Part print with two shaded views. Sizes in mm from the minimum x, y, z corner. A direction names the side the tool comes from. Round coordinates to 2 decimals unless told otherwise and drop trailing zeros. Order: outer loops, then holes, each group sorted by start corner. A loop starts at its lowest first (then second) coordinate and runs counter-clockwise, first axis right, second up. Notation, with made-up numbers: M 83.5,33 L 131.5,33 A12 cw 131.5,37 Z; hole C 37.5,83 d3. An arc over 180 degrees is marked long. Return JSON: item names as keys, results as strings. Group by question number.
Item 1: Pull direction X, two halves, no side cores. Call the marked faces 1, 2 and 3: pulls with the +X half, pulls with the -X half, needs draft (parallel to the pull), parting line crosses it, or undercut.
Item 2: Slice it at D-D on y = 24. Write the cut outline in (x, z) (3 decimals), then the cut area to 3 significant figures.
Item 3: Pin check, flat tips, straight feed: pin 1 Ø3.5 at (x, y) = (14, 4) entering from -Z; pin 2 Ø6 at (x, y) = (12.5, 12) entering from -Z; pin 3 Ø2 at (y, z) = (6.5, 2.5) entering from -X; pin 4 Ø1 at (y, z) = (24, 4.5) entering from +X. Stop position of each tip, or through.
Item 4: Which spindle directions (+Z, -Z, +X, -X, +Y, -Y) get a long thin tool onto all of the face, cutting with end or side? Do the marked faces 4 and 5. Say none if no direction does.
Item 5: Slice it at A-A on y = 14. Write the cut outline in (x, z) (3 decimals).
Item 6: Probe line 1 along Y through (x, z) = (14, 2.6) (3 decimals); line 2 along Z through (x, y) = (26.75, 14.5); line 3 along X through (y, z) = (4, 3.35) (3 decimals). List the from-to ranges inside material, lowest first.
Item 7: Slice it at C-C on z = 0.95. Write the cut outline in (x, y) (3 decimals), then the cut area to 3 significant figures.
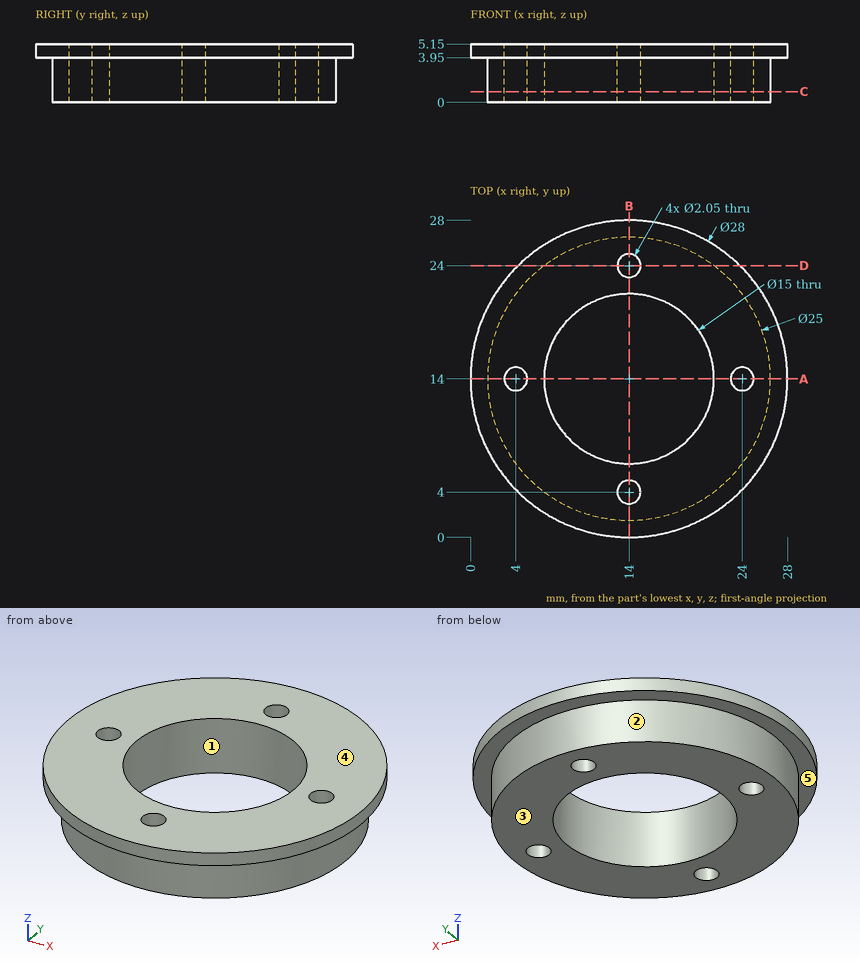
Output values:
{
 "1": {"face 1": "undercut", "face 2": "parting line crosses it", "face 3": "needs draft"},
 "2": {"outline": "M 4.202,3.95 L 6.5,3.95 L 6.5,0 L 12.975,0 L 12.975,5.15 L 4.202,5.15 Z; M 15.025,0 L 21.5,0 L 21.5,3.95 L 23.798,3.95 L 23.798,5.15 L 15.025,5.15 Z", "area": "72.2 mm²"},
 "3": {"pin 1": "z = 0", "pin 2": "through", "pin 3": "x = 3.32", "pin 4": "x = 24.28"},
 "4": {"face 4": "+Z, +X, -X, +Y, -Y", "face 5": "-Z"},
 "5": {"outline": "M 0,3.95 L 1.5,3.95 L 1.5,0 L 2.975,0 L 2.975,5.15 L 0,5.15 Z; M 5.025,0 L 6.5,0 L 6.5,5.15 L 5.025,5.15 Z; M 21.5,0 L 22.975,0 L 22.975,5.15 L 21.5,5.15 Z; M 25.025,0 L 26.5,0 L 26.5,3.95 L 28,3.95 L 28,5.15 L 25.025,5.15 Z"},
 "6": {"line 1": "1.5 to 2.975, 5.025 to 6.5, 21.5 to 22.975, 25.025 to 26.5", "line 2": "3.95 to 5.15", "line 3": "6.5 to 12.975, 15.025 to 21.5"},
 "7": {"outline": "C 14,14 d25; hole C 4,14 d2.05; hole C 14,14 d15; hole C 14,4 d2.05; hole C 14,24 d2.05; hole C 24,14 d2.05", "area": "301 mm²"}
}
